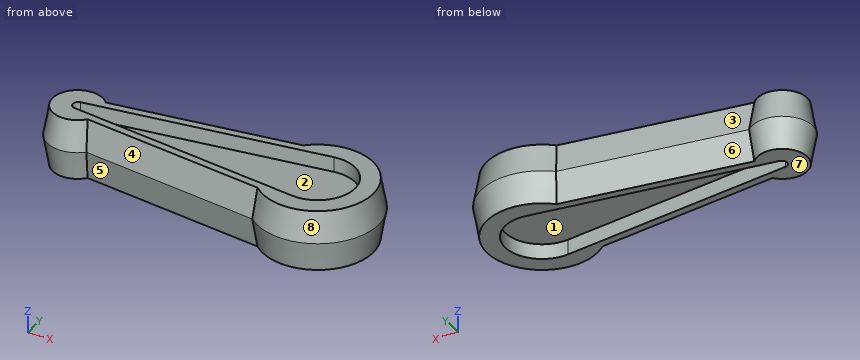
Autodesk Inventor part; units mm, degrees
ref_plane "YZ Plane" through (0, 0, 0) normal (1, 0, 0) x (0, 1, 0)
ref_plane "XZ Plane" through (0, 0, 0) normal (0, 1, 0) x (-1, 0, 0)
ref_plane "XY Plane" through (0, 0, 0) normal (0, 0, 1) x (1, 0, 0)
sketch "Sketch1" plane through (0, 0, 0) normal (0, 0, 1) x (1, 0, 0)
  line L0 (-40.64, 0) -> (154.94, 0)
  line L1 (0, -35.56) -> (0, 35.56)
  arc A0 (8.901936, 9.057899) -> (8.901936, -9.057899) centre (0, 0) ccw
  arc A1 (84.799479, -19.05) -> (84.799479, 19.05) centre (101.6, 0) ccw
  line L2 (8.901936, 9.057899) -> (84.799479, 19.05)
  line L3 (8.901936, -9.057899) -> (84.799479, -19.05)
  dimension "d1" = 25.4
  dimension "d3" = 50.8
  dimension "d4" = 15
  dimension "d5" = 38.1
  dimension "d6" = 101.6
sketch "Sketch1 outline for Extrusion1" plane through (0, 0, 0) normal (0, 0, 1) x (1, 0, 0)
  arc A0 (8.901936, 9.057899) -> (8.901936, -9.057899) centre (0, 0) ccw
  line L0 (84.799479, 19.05) -> (8.901936, 9.057899)
  arc A1 (84.799479, -19.05) -> (84.799479, 19.05) centre (101.6, 0) ccw
  line L1 (8.901936, -9.057899) -> (84.799479, -19.05)
extrude "Extrusion1" add sketch "Sketch1 outline for Extrusion1" along normal mid plane 25.4 draft -10
sketch "Sketch2" plane through (0, 0, 12.7) normal (0, 0, 1) x (1, 0, 0)
  line L0 (0, 2.296768) -> (99.571808, 15.405645)
  line L1 (8.044726, 6.686369) -> (85.785782, 16.921173)
  line L2 (0, -35.56) -> (0, 35.56)
  line L3 (-40.64, 0) -> (154.94, 0)
  line L4 (0, -2.296768) -> (99.571808, -15.405645)
  arc A0 (0, 2.296768) -> (0, -2.296768) centre (0.302375, 0) ccw
  arc A1 (99.571808, -15.405645) -> (99.571808, 15.405645) centre (101.6, 0) ccw
  arc A2 (85.785782, -16.921173) -> (85.785782, 16.921173) centre (101.6, 0) ccw
  point P0 (0, 0)
  point P1 (8.355059, 3.396732)
  point P2 (8.355059, -3.396732)
  dimension "d10" = 3.302
extrude "Extrusion2" cut sketch "Sketch2" against normal blind 6.35
sketch "Sketch3" plane through (0, 0, -12.7) normal (0, 0, -1) x (-1, 0, 0)
  arc A0 (0, -2.296768) -> (0, 2.296768) centre (-0.302375, 0) ccw
  arc A1 (0, -2.296768) -> (0, 2.296768) centre (-0.302375, 0) ccw
  line L0 (-99.571808, -15.405645) -> (0, -2.296768)
  line L1 (0, 2.296768) -> (-99.571808, 15.405645)
  arc A2 (-99.571808, 15.405645) -> (-99.571808, -15.405645) centre (-101.6, 0) ccw
  arc A3 (-99.571808, 15.405645) -> (-99.571808, -15.405645) centre (-101.6, 0) ccw
  line L2 (0, -2.296768) -> (-99.571808, -15.405645)
  line L3 (-85.785782, 16.921173) -> (-8.044726, 6.686369)
  point P0 (0, 0)
  point P1 (0, 2.296768)
extrude "Extrusion3" cut sketch "Sketch3" against normal blind 6.35
properties part number "Ch3 Part 2"
Work out the finished part from the listing and answer in its coordinate system (mm). Face numbers are marked on the shaded views. A direction names the side the tool comes from. Round coordinates to 2 decimals unless told otherwise and drop trailing zeros. Order: outer loops, then holes, each group sorted by start corner. A loop starts at its lowest first (then second) coordinate and runs counter-clockwise, first axis right, second up.
Q1. A cutting plane is placed at A-A, the plane x = 101.6. Determine the outline of the cut face in (y, z).
Solution:
outline: (-25.4, 0) - (-23.16, -12.7) - (-15.54, -12.7) - (-15.54, -6.35) - (15.54, -6.35) - (15.54, -12.7) - (23.16, -12.7) - (25.4, 0) - (23.16, 12.7) - (15.54, 12.7) - (15.54, 6.35) - (-15.54, 6.35) - (-15.54, 12.7) - (-23.16, 12.7) - close
Q2. Given pin 1 Ø3 at (x, y) = (23.5, -3) entering from -Z; pin 2 Ø18.5 at (x, y) = (101.6, 0) entering from +Z; pin 3 Ø2 at (x, z) = (37.5, 3.5) entering from +Y, each flat-ended and moving along its own axis, determine where each tip first touches the part or whether it passes through.
Solution:
pin 1: stops at z = -6.35
pin 2: stops at z = 6.35
pin 3: stops at y = 12.42
Q3. A cutting plane is placed at D-D, the plane z = 2.75. Determine the outline of the cut face in (x, y), then the cut area to 3 significant figures.
Solution:
outline: (8.73, -8.55) - (85.01, -18.59) arc R24.92 ccw (long way) to (85.01, 18.59) - (8.73, 8.55) arc R12.22 ccw (long way) to start
area: 4,230 mm2
Q4. A cutting plane is placed at C-C, the plane z = 8.75. Determine the outline of the cut face in (x, y), then the cut area to 3 significant figures.
Solution:
outline: (8.33, -7.43) - (85.48, -17.58) arc R23.86 ccw (long way) to (85.48, 17.58) - (8.33, 7.43) arc R11.16 ccw (long way) to start; hole (0, -2.3) - (99.57, -15.41) arc R15.54 ccw (long way) to (99.57, 15.41) - (0, 2.3) arc R2.32 ccw to start
area: 1,680 mm2
Q5. The mould has two halves that part along X. Classify the marked faces 5, 6, 7 and 8: pulls with the +X half, pulls with the -X half, needs draft (parallel to the pull), parting line crosses it, or undercut.
Solution:
face 5: undercut
face 6: undercut
face 7: needs draft
face 8: parting line crosses it
Q6. A cutting plane is placed at B-B, the plane y = 0. Determine the outline of the cut face in (x, z).
Solution:
outline: (-12.7, 0) - (-10.46, -12.7) - (-2.01, -12.7) - (-2.01, -6.35) - (117.14, -6.35) - (117.14, -12.7) - (124.76, -12.7) - (127, 0) - (124.76, 12.7) - (117.14, 12.7) - (117.14, 6.35) - (-2.01, 6.35) - (-2.01, 12.7) - (-10.46, 12.7) - close
Q7. Find the intervals of material crossed by line 1 along Z through (x, y) = (70.5, 8.5); line 2 along Y through (x, z) = (101.6, -7.25); line 3 along Y through (x, z) = (102.5, 9.5), in increasing order.
Solution:
line 1: z = -6.35 to 6.35
line 2: y = -24.12 to -15.54, 15.54 to 24.12
line 3: y = -23.71 to -15.51, 15.51 to 23.71
Q8. A tool of negligible diameter and unlimited length cuts with its end or side. For the marked faces 1, 2, 3 and 4, from which of +Z, -Z, +X, -X, +Y, -Y can it reach the whole face along a straight path? Write none if from no direction.
Solution:
face 1: -Z
face 2: +Z
face 3: +Z, +Y
face 4: +Z, -Y
